For this review, take the finished solid that the model builds, in its own axes (mm). Give positions to 0.01 mm unless a question says otherwise; leave off trailing zeros. Order: outer loops, then holes, each group sorted by start corner. A loop starts at its lowest first (then second) coordinate and runs counter-clockwise, first axis right, second up.
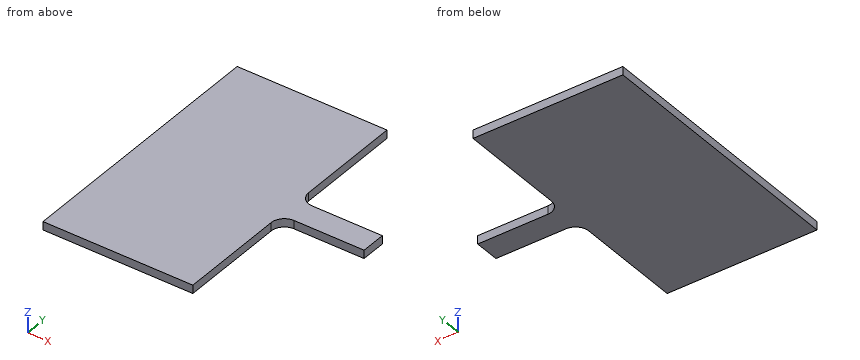
from build123d import *

# Parameters (mm, degrees)
BOSS_EXTRUDE1_DEPTH = 1


with BuildPart() as part:
    # Sketch1 → Boss-Extrude1 (new body)
    with BuildSketch(Plane.XY):
        with BuildLine():
            Line((29.736292646, -7), (11.736292646, -7))
            Line((11.736292646, -7), (11.736292646, 25))
            Line((11.736292646, 25), (29.736292646, 25))
            Line((29.736292646, 25), (29.736292646, 12.0875))
            ThreePointArc((29.736292646, 12.0875), (30.201260631, 10.964967985), (31.323792646, 10.5))
            Line((31.323792646, 10.5), (39.736292646, 10.5))
            Line((39.736292646, 10.5), (39.736292646, 7.5))
            Line((39.736292646, 7.5), (31.323792646, 7.5))
            ThreePointArc((31.323792646, 7.5), (30.201260631, 7.035032015), (29.736292646, 5.9125))
            Line((29.736292646, 5.9125), (29.736292646, -7))
        make_face()
    extrude(amount=BOSS_EXTRUDE1_DEPTH)


solid = part.part
1) We need section A-A on z = 0.6. Give the boundary of the cut face in (x, y) (1 decimal).
Answer sheet:
outline: (11.7, -7) - (29.7, -7) - (29.7, 5.9) arc R1.6 cw to (31.3, 7.5) - (39.7, 7.5) - (39.7, 10.5) - (31.3, 10.5) arc R1.6 cw to (29.7, 12.1) - (29.7, 25) - (11.7, 25) - close
2) We need section C-C on x = 30.5. Give the boundary of the cut face in (y, z), then the cut area to 3 significant figures.
Answer sheet:
outline: (7.27, 0) - (10.73, 0) - (10.73, 1) - (7.27, 1) - close
area: 3.46 mm2
3) We need section B-B on y = 1.5. Give the boundary of the cut face in (x, z).
Answer sheet:
outline: (11.74, 0) - (29.74, 0) - (29.74, 1) - (11.74, 1) - close
4) To check wall thickness, follow line 1 (Y direction, x = 33.5, z = 0.75); line 2 (X direction, y = 16, z = 0.4); line 3 (X direction, y = 7, z = 0.8). State the ranges of each line that lie inside material, in increasing order.
Answer sheet:
line 1: y = 7.5 to 10.5
line 2: x = 11.74 to 29.74
line 3: x = 11.74 to 30.17
